Input: part model. Units: mm. Frame: model coordinates. Face numbers are marked on the shaded views. A direction names the side the tool comes from. Coordinates: 2 decimals unless noted, no trailing zeros. Loops run counter-clockwise (first coordinate to the right, second up) from the corner with the lowest first, then second, coordinate; pieces in that order, holes last. Notation, with made-up numbers: (-28, -1) - (13, -1) arc R28 ccw to (13, 19) - close; hole circle Ø11 at (52.5, 0). An arc over 180 degrees is marked (long way). Answer as CSV lines item,"result". Start each with the question number.
```python
from build123d import *

# Parameters (mm, degrees)
BOSS_EXTRUDE1_DEPTH = 10
SKETCH2_R           = 1.5
CUT_EXTRUDE1_DEPTH  = 40.761790704
SKETCH3_R           = 1.5
CUT_EXTRUDE2_DEPTH  = 40.761790704


with BuildPart() as part:
    # Sketch1 → Boss-Extrude1 (new body)
    with BuildSketch(Plane(origin=(0, 0, 0), x_dir=(1, 0, 0), z_dir=(0, 1, 0))):
        with BuildLine():
            Line((-8, -15), (-8, 35))
            Line((-8, 35), (-3.5, 35))
            Line((-3.5, 35), (-3.5, 7.193747285))
            ThreePointArc((-3.5, 7.193747285), (4.242640687, 6.782329983), (8, 0))
            Line((8, 0), (8, -15))
            Line((8, -15), (3.5, -15))
            Line((3.5, -15), (3.5, -1.720465053))
            ThreePointArc((3.5, -1.720465053), (0, 3.9), (-3.5, -1.720465053))
            Line((-3.5, -1.720465053), (-3.5, -15))
            Line((-3.5, -15), (-8, -15))
        make_face()
    extrude(amount=BOSS_EXTRUDE1_DEPTH)

    # Sketch2 → Cut-Extrude1 (cut, through all)
    with BuildSketch(Plane.ZY.offset(8)):
        with Locations((10, 5)):
            Circle(SKETCH2_R)
    extrude(amount=-CUT_EXTRUDE1_DEPTH, mode=Mode.SUBTRACT)

    # Sketch3 → Cut-Extrude2 (cut, through all)
    with BuildSketch(Plane.ZY.offset(8)):
        with Locations((-24, 7)):
            Circle(SKETCH3_R)
        with Locations((-15, 7)):
            Circle(SKETCH3_R)
    extrude(amount=-CUT_EXTRUDE2_DEPTH, mode=Mode.SUBTRACT)


solid = part.part
```
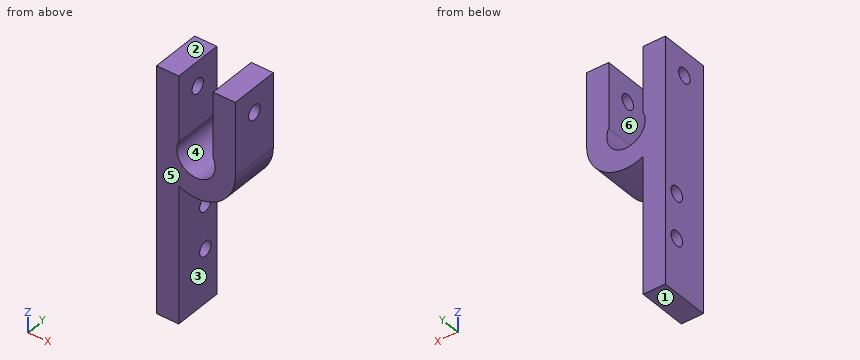
Item 1: Section query B-B, the plane y = 7. Output: boundary loops of the cut face in (x, z).
Item 2: Material intervals for probe 1 along X at (y, z) = (8.75, 5); probe 2 along X at (y, z) = (1.5, 0); probe 3 along Y at (x, z) = (-6.5, -15), sorted ascending.
Item 3: Section query D-D, the plane y = 9. Output: boundary loops of the cut face in (x, z).
Item 4: Draft query along Z for the marked faces 1, 2, 3 and 4. Return one class per face: pulls with the +Z half, pulls with the -Z half, needs draft (parallel to the pull), parting line crosses it, or undercut.
Item 5: Section query C-C, the plane z = 10. Output: boundary loops of the cut face in (x, y), and give its area (3 significant figures).
Item 6: Contact query for flat-ended pins moving along their axis: P1, Ø2.5, axis at y = 7, z = -24, coming from the -X side; P2, Ø6, axis at y = 6, z = -6.5, coming from the +X side; P3, Ø5, axis at y = 5, z = 10, coming from the +X side. Output: stop coordinate, or through.
Item 7: Section query A-A, the plane z = 4.5. Output: boundary loops of the cut face in (x, y).
Item 8: Set-up query: the marked faces 5 and 6. Return all of +Z, -Z, +X, -X, +Y, -Y with unobstructed straight access to the full face (end or side cutting, diameter ignored); none if empty.
Response values:
1,outline,"(-8, -35) - (-3.5, -35) - (-3.5, -25.5) - (-8, -25.5) - close; (-8, -22.5) - (-3.5, -22.5) - (-3.5, -16.5) - (-8, -16.5) - close; (-8, -13.5) - (-3.5, -13.5) - (-3.5, -7.19) arc R8 ccw to (8, 0) - (8, 15) - (3.5, 15) - (3.5, 1.72) arc R3.9 cw (long way) to (-3.5, 1.72) - (-3.5, 15) - (-8, 15) - close"
2,probe 1,"x = -8 to -3.5, 3.5 to 8"
2,probe 2,"x = -8 to -3.9, 3.9 to 8"
2,probe 3,"y = 0 to 5.5, 8.5 to 10"
3,outline,"(-8, -35) - (-3.5, -35) - (-3.5, -7.19) arc R8 ccw to (8, 0) - (8, 15) - (3.5, 15) - (3.5, 1.72) arc R3.9 cw (long way) to (-3.5, 1.72) - (-3.5, 15) - (-8, 15) - close"
4,face 1,"pulls with the -Z half"
4,face 2,"pulls with the +Z half"
4,face 3,"needs draft"
4,face 4,"undercut"
5,outline,"(-8, 0) - (-3.5, 0) - (-3.5, 3.5) - (-8, 3.5) - close; (-8, 6.5) - (-3.5, 6.5) - (-3.5, 10) - (-8, 10) - close; (3.5, 0) - (8, 0) - (8, 3.5) - (3.5, 3.5) - close; (3.5, 6.5) - (8, 6.5) - (8, 10) - (3.5, 10) - close"
5,area,"63.0 mm²"
6,P1,"passes through"
6,P2,"stops at x = 7.19"
6,P3,"stops at x = 8"
7,outline,"(-8, 0) - (-3.5, 0) - (-3.5, 10) - (-8, 10) - close; (3.5, 0) - (8, 0) - (8, 10) - (3.5, 10) - close"
8,face 5,"+Z, -Z, +X, -X, -Y"
8,face 6,"+Z, +Y, -Y"
